from build123d import *


with BuildPart() as part:
    # Croquis1 → Revolución1 (revolve)
    with BuildSketch(Plane(origin=(0, 0, 0), x_dir=(0, 0, -1), z_dir=(1, 0, 0))):
        Polygon((54.267285515, 67.95416726), (54.267285515, -66.513442866), (128.224471084, -66.513442866), (128.224471084, -60.270303824), (128.224471084, 59.309820895), (133.507127196, 59.309820895), (133.507127196, 67.95416726), align=None)
        Polygon((128.224471084, -60.270303824), (128.224471084, -66.513442866), (128.224471084, -71.796098978), (133.507127196, -66.513442866), (133.507127196, -60.270303824), align=None)
    revolve(axis=Axis((0, -66.513442866, 0), (0, 1, 0)))


solid = part.part
CAD build for the part. Positions are in the model's coordinates, mm. A direction names the side the tool comes from. Coordinates: 2 decimals unless noted, no trailing zeros. Loops run counter-clockwise (first coordinate to the right, second up) from the corner with the lowest first, then second, coordinate; pieces in that order, holes last. Notation, with made-up numbers: (84, -39.75) - (89, -39.75) arc R13 cw to (89, -14.75) - close; hole circle Ø6 at (-12, -24.5). An arc over 180 degrees is marked (long way). Write item = value, one per line. Start each with the question number.
Q1. Drill centre lines: L1, parallel to X at y = 26, z = 0; L2, parallel to Y at x = -113.5, z = 59. Where is each one in solid material? Low to high.
Q2. Pull direction Y, two halves, no side cores. Call faces 1 (the flat face through (-119, 59.31, -50)), 2 (the flat face through (-2, 67.954, -57)), 3 (the cylindrical face through (-132.37, 63.69, 17.38)), 4 (the cylindrical face through (125.175, 0.357, 27.797)): pulls with the +Y half, pulls with the -Y half, needs draft (parallel to the pull), parting line crosses it, or undercut.
Q3. Which spindle directions (+Z, -Z, +X, -X, +Y, -Y) get a long thin tool onto all of the face, cutting with end or side? Do faces 5 (the flat face through (-119, -60.27, 50)), 6 (the cylindrical face through (-132.37, -63.35, 17.38)), 7 (the flat face through (-2, -66.513, 55)). Say none if no direction does.
Q4. Cut at B-B, the plane z = 0. List the corners of the cut face in (x, y), then the cut area to 3 significant figures.
Q5. Flat gauge pins, fed straight in: pin 1 Ø1.5 at (y, z) = (-57, -82) entering from -X; pin 2 Ø5 at (x, y) = (84, 44.5) entering from +Z; pin 3 Ø1 at (y, z) = (31.5, 29.5) entering from +X. Where does each tip first touch, or does it go through?
Q6. Cut at C-C, the plane y = 8. List the corners of the cut face in (x, z).
Q7. Cut at A-A, the plane x = 0. List the corners of the cut face in (y, z), then the cut area to 3 significant figures.
Computed:
q1.L1 = -128.22 to -54.27, 54.27 to 128.22
q1.L2 = -66.51 to 67.95
q2.face_1 = undercut
q2.face_2 = pulls with the +Y half
q2.face_3 = needs draft
q2.face_4 = undercut
q3.face_5 = none
q3.face_6 = +Y, -Y
q3.face_7 = -Y
q4.outline = (-133.51, -66.51) - (-128.22, -71.8) - (-128.22, -66.51) - (-54.27, -66.51) - (-54.27, 67.95) - (-133.51, 67.95) - (-133.51, 59.31) - (-128.22, 59.31) - (-128.22, -60.27) - (-133.51, -60.27) - close; (54.27, -66.51) - (128.22, -66.51) - (128.22, -71.8) - (133.51, -66.51) - (133.51, -60.27) - (128.22, -60.27) - (128.22, 59.31) - (133.51, 59.31) - (133.51, 67.95) - (54.27, 67.95) - close
q4.area = 20,100 mm²
q5.pin_1 = -99.2
q5.pin_2 = 98.99
q5.pin_3 = 124.9
q6.outline = circle Ø256.45 at (0, 0); hole circle Ø108.53 at (0, 0)
q7.outline = (-71.8, -128.22) - (-66.51, -133.51) - (-60.27, -133.51) - (-60.27, -128.22) - (59.31, -128.22) - (59.31, -133.51) - (67.95, -133.51) - (67.95, -54.27) - (-66.51, -54.27) - (-66.51, -128.22) - close; (-71.8, 128.22) - (-66.51, 128.22) - (-66.51, 54.27) - (67.95, 54.27) - (67.95, 133.51) - (59.31, 133.51) - (59.31, 128.22) - (-60.27, 128.22) - (-60.27, 133.51) - (-66.51, 133.51) - close
q7.area = 20,100 mm²
